Model file for the job. Use its own axes, mm. Face numbers are marked on the shaded views. A direction names the side the tool comes from. Coordinates: 2 decimals unless noted, no trailing zeros. Write each loop counter-clockwise with the first axis right and the second up, starting at its lowest first coordinate (ties: lowest second). Pieces come first, ordered by that corner, then holes. Notation, with made-up numbers: (54, 36.25) - (66, 36.25) arc R35 ccw to (66, 72.25) - close; hole circle Ø10 at (-37, -8). An arc over 180 degrees is marked (long way). Put each result on its own line as item: value. Start each with the question number.
1. Saw through at A-A, the plane z = 4.3. Write the cut outline in (x, y), plus the area to 3 significant figures.
2. Saw through at D-D, the plane y = -9.5. Give the number of separate pieces and of enclosed holes in the cut face, plus the area to 3 significant figures.
3. Saw through at B-B, the plane x = -2. Write the cut outline in (y, z), plus the area to 3 significant figures.
4. Drop flat-ended pins along their axis: P1, Ø1.9, axis at x = -0.5, y = 17.5, coming from the +Z side; P2, Ø2, axis at x = -8, y = -8.5, coming from the +Z side; P3, Ø1.2, axis at x = 1.5, z = 4, coming from the +Y side; P4, Ø2, axis at y = 18.5, z = 3.5, coming from the -X side. Give the stop position or say it passes through.
5. Pull direction Y, two halves, no side cores. Call the marked faces 1, 2, 3 and 4: released by +Y, released by -Y, zero draft, split by the parting line, or undercut.
6. Drill centre lines: L1, parallel to X at y = 0, z = 1.95; L2, parallel to Y at x = -6, z = 3.3; L3, parallel to Y at x = 7.25, z = 1.95. Where is each one in solid material? Low to high. Write a range as from..to.
7. Saw through at C-C, the plane y = -2. Write the cut outline in (x, z), plus the area to 3 significant figures.
8. Which spindle directions (+Z, -Z, +X, -X, +Y, -Y) get a long thin tool onto all of the face, cutting with end or side? Do the marked faces 5, 6 and 7. Say none if no direction does.
```python
from build123d import *

# Parameters (mm, degrees)
SKETCH_R        = 7
SKETCH_R_2      = 1.7
PAD_DEPTH       = 5
SKETCH001_R     = 8.5
SKETCH001_W     = 6.2
SKETCH001_H     = 20
POCKET_DEPTH    = 2.5
FILLET_R        = 4
FILLET001_R     = 4
FILLET002_R     = 4
FILLET003_R     = 4
FILLET004_R     = 4
FILLET005_R     = 4
FILLET006_R     = 1
CHAMFER_SIZE    = 1.5
CHAMFER001_SIZE = 1.5
CHAMFER002_SIZE = 1.5
CHAMFER003_SIZE = 1.5
CHAMFER004_SIZE = 1.5
CHAMFER005_SIZE = 1.7


with BuildPart() as part:
    # Sketch → Pad (new body)
    with BuildSketch(Plane.XY):
        Polygon((-12.5, -12.5), (12.5, -12.5), (12.5, 12.5), (9, 25.5), (-9, 25.5), (-12.5, 12.5), align=None)
        Circle(SKETCH_R, mode=Mode.SUBTRACT)
        with Locations((-8, 8.5)):
            Circle(SKETCH_R_2, mode=Mode.SUBTRACT)
        with Locations((8, 8.5)):
            Circle(SKETCH_R_2, mode=Mode.SUBTRACT)
        with Locations((-8, -8.5)):
            Circle(SKETCH_R_2, mode=Mode.SUBTRACT)
        with Locations((8, -8.5)):
            Circle(SKETCH_R_2, mode=Mode.SUBTRACT)
        with Locations((-6, 20)):
            Circle(SKETCH_R_2, mode=Mode.SUBTRACT)
        with Locations((6, 20)):
            Circle(SKETCH_R_2, mode=Mode.SUBTRACT)
    extrude(amount=PAD_DEPTH)

    # Sketch001 → Pocket (cut)
    with BuildSketch(Plane.XY.offset(5)):
        Circle(SKETCH001_R)
        with Locations((0, 20)):
            Rectangle(SKETCH001_W, SKETCH001_H)
    extrude(amount=-POCKET_DEPTH, mode=Mode.SUBTRACT)

    # Fillet
    fillet_edges = [part.edges().sort_by_distance(p)[0] for p in [
        (-12.5, -12.5, 2.5),
    ]]
    fillet(fillet_edges, radius=FILLET_R)

    # Fillet001
    fillet001_edges = [part.edges().sort_by_distance(p)[0] for p in [
        (12.5, -12.5, 2.5),
    ]]
    fillet(fillet001_edges, radius=FILLET001_R)

    # Fillet002
    fillet002_edges = [part.edges().sort_by_distance(p)[0] for p in [
        (-12.5, 12.5, 2.5),
    ]]
    fillet(fillet002_edges, radius=FILLET002_R)

    # Fillet003
    fillet003_edges = [part.edges().sort_by_distance(p)[0] for p in [
        (12.5, 12.5, 2.5),
    ]]
    fillet(fillet003_edges, radius=FILLET003_R)

    # Fillet004
    fillet004_edges = [part.edges().sort_by_distance(p)[0] for p in [
        (9, 25.5, 2.5),
    ]]
    fillet(fillet004_edges, radius=FILLET004_R)

    # Fillet005
    fillet005_edges = [part.edges().sort_by_distance(p)[0] for p in [
        (-9, 25.5, 2.5),
    ]]
    fillet(fillet005_edges, radius=FILLET005_R)

    # Fillet006
    fillet006_edges = [part.edges().sort_by_distance(p)[0] for p in [
        (0, 25.5, 0),
    ]]
    fillet(fillet006_edges, radius=FILLET006_R)

    # Chamfer
    chamfer_edges = [part.edges().sort_by_distance(p)[0] for p in [
        (-9.7, -8.5, 0),
    ]]
    chamfer(chamfer_edges, length=CHAMFER_SIZE)

    # Chamfer001
    chamfer001_edges = [part.edges().sort_by_distance(p)[0] for p in [
        (-9.7, 8.5, 0),
    ]]
    chamfer(chamfer001_edges, length=CHAMFER001_SIZE)

    # Chamfer002
    chamfer002_edges = [part.edges().sort_by_distance(p)[0] for p in [
        (6.3, -8.5, 0),
    ]]
    chamfer(chamfer002_edges, length=CHAMFER002_SIZE)

    # Chamfer003
    chamfer003_edges = [part.edges().sort_by_distance(p)[0] for p in [
        (6.3, 8.5, 0),
    ]]
    chamfer(chamfer003_edges, length=CHAMFER003_SIZE)

    # Chamfer004
    chamfer004_edges = [part.edges().sort_by_distance(p)[0] for p in [
        (-7.7, 20, 0),
    ]]
    chamfer(chamfer004_edges, length=CHAMFER004_SIZE)

    # Chamfer005
    chamfer005_edges = [part.edges().sort_by_distance(p)[0] for p in [
        (4.3, 20, 0),
    ]]
    chamfer(chamfer005_edges, length=CHAMFER005_SIZE)


solid = part.part
```
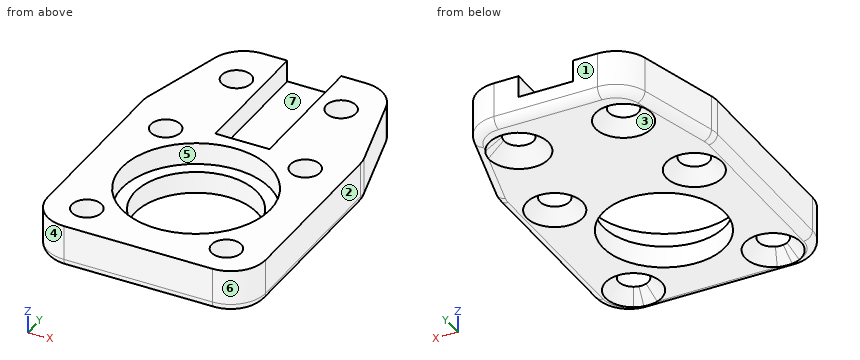
Final values:
1. outline: (-12.5, -8.5) arc R4 ccw to (-8.5, -12.5) - (8.5, -12.5) arc R4 ccw to (12.5, -8.5) - (12.5, 11.97) arc R4 ccw to (12.36, 13.01) - (9.8, 22.54) arc R4 ccw to (5.93, 25.5) - (3.1, 25.5) - (3.1, 10) - (-3.1, 10) - (-3.1, 25.5) - (-5.93, 25.5) arc R4 ccw to (-9.8, 22.54) - (-12.36, 13.01) arc R4 ccw to (-12.5, 11.97) - close; hole circle Ø3.4 at (-8, -8.5); hole circle Ø3.4 at (-8, 8.5); hole circle Ø17 at (0, 0); hole circle Ø3.4 at (-6, 20); hole circle Ø3.4 at (6, 20); hole circle Ø3.4 at (8, -8.5); hole circle Ø3.4 at (8, 8.5)
1. area: 516 mm²
2. separate pieces: 3
2. enclosed holes: 0
2. area: 90.7 mm²
3. outline: (-12.5, 1) arc R1 ccw to (-11.5, 0) - (-6.71, 0) - (-6.71, 2.5) - (-8.26, 2.5) - (-8.26, 5) - (-12.5, 5) - close; (6.71, 0) - (24.5, 0) arc R1 ccw to (25.5, 1) - (25.5, 2.5) - (10, 2.5) - (10, 5) - (8.26, 5) - (8.26, 2.5) - (6.71, 2.5) - close
3. area: 76.0 mm²
4. P1: stops at z = 2.5
4. P2: passes through
4. P3: stops at y = 10
4. P4: stops at x = -11.15
5. face 1: released by +Y
5. face 2: zero draft
5. face 3: undercut
5. face 4: released by -Y
6. L1: x = -12.5..-7, 7..12.5
6. L2: y = -12.5..-6.02, 6.02..18.3, 21.7..25.5
6. L3: y = -12.5..-10.03, -6.97..6.97, 10.03..18.85, 21.15..25.28
7. outline: (-12.5, 1) arc R1 ccw to (-11.5, 0) - (-6.71, 0) - (-6.71, 2.5) - (-8.26, 2.5) - (-8.26, 5) - (-12.5, 5) - close; (6.71, 0) - (11.5, 0) arc R1 ccw to (12.5, 1) - (12.5, 5) - (8.26, 5) - (8.26, 2.5) - (6.71, 2.5) - close
7. area: 49.7 mm²
8. face 5: +Z
8. face 6: +Z, -Z, +X, -Y
8. face 7: +Z, +Y
